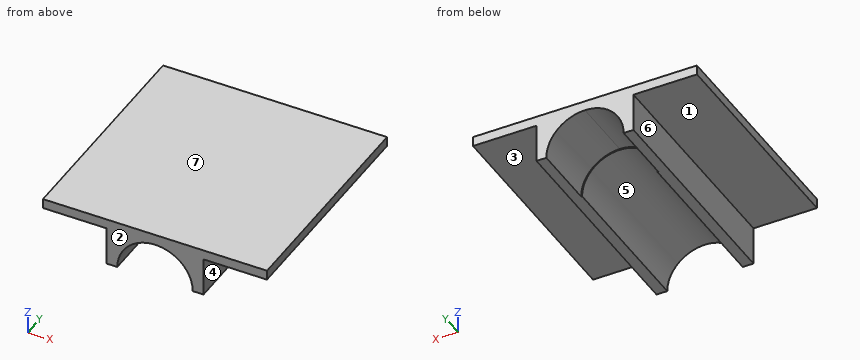
from build123d import *

# Parameters (mm, degrees)
BOSS_EXTRUDE4_DEPTH = 51.39
BOSS_EXTRUDE5_DEPTH = 72.39


with BuildPart() as part:
    # Sketch1 → Boss-Extrude4 (new body)
    with BuildSketch(Plane(origin=(0, 0, 0), x_dir=(1, 0, 0), z_dir=(0, 1, 0))):
        with BuildLine():
            ThreePointArc((18.7283116, 30.198170271), (6.5283116, 17.99817027), (-5.6716884, 30.198170271))
            Line((-5.6716884, 30.198170271), (-9.146688396, 30.198170271))
            Line((-9.146688396, 30.198170271), (-9.146688396, 17.698170271))
            Line((-9.146688396, 17.698170271), (-29.681604426, 17.698170271))
            Line((-29.681604426, 17.698170271), (-29.681604426, 14.523170271))
            Line((-29.681604426, 14.523170271), (42.719057074, 14.523170271))
            Line((42.719057074, 14.523170271), (42.719057074, 17.698170271))
            Line((42.719057074, 17.698170271), (22.203311604, 17.698170271))
            Line((22.203311604, 17.698170271), (22.203311604, 30.198170271))
            Line((22.203311604, 30.198170271), (18.7283116, 30.198170271))
        make_face()
    extrude(amount=BOSS_EXTRUDE4_DEPTH)

    # Sketch1_9 → Boss-Extrude5 (add)
    with BuildSketch(Plane(origin=(0, 0, 0), x_dir=(1, 0, 0), z_dir=(0, 1, 0))):
        Polygon((22.203311604, 17.698170271), (6.528311562, 17.698170271), (-9.146688396, 17.698170271), (-29.681604426, 17.698170271), (-29.681604426, 14.523170271), (42.719057074, 14.523170271), (42.719057074, 17.698170271), align=None)
        with BuildLine():
            ThreePointArc((19.028311604, 30.198170271), (15.367146354, 21.359335491), (6.528311562, 17.698170271))
            Line((6.528311562, 17.698170271), (22.203311604, 17.698170271))
            Line((22.203311604, 17.698170271), (22.203311604, 30.198170271))
            Line((22.203311604, 30.198170271), (19.028311604, 30.198170271))
        make_face()
        with BuildLine():
            ThreePointArc((6.528311562, 17.698170271), (-2.310523175, 21.359335521), (-5.971688396, 30.198170271))
            Line((-5.971688396, 30.198170271), (-9.146688396, 30.198170271))
            Line((-9.146688396, 30.198170271), (-9.146688396, 17.698170271))
            Line((-9.146688396, 17.698170271), (6.528311562, 17.698170271))
        make_face()
    extrude(amount=BOSS_EXTRUDE5_DEPTH)


solid = part.part
Design review of the part built by this model. Coordinates are the model's own, in mm. Face numbers are marked on the shaded views. A direction names the side the tool comes from. Give positions to 0.01 mm unless a question says otherwise; leave off trailing zeros. Order: outer loops, then holes, each group sorted by start corner. A loop starts at its lowest first (then second) coordinate and runs counter-clockwise, first axis right, second up. Notation, with made-up numbers: (-13.75, 34) - (28.25, 34) arc R17 cw to (28.25, 57) - close; hole circle Ø4 at (28, -21.5). An arc over 180 degrees is marked (long way). Write item = value, one per line. Start each with the question number.
Q1. To check wall thickness, follow L1, parallel to Z at x = -21.5, y = 7; L2, parallel to X at y = 21, z = -23.5; L3, parallel to X at y = 52, z = -20.5. State the ranges of each line that lie inside material, in increasing order. Write a range as from..to.
Q2. We need section C-C on z = -20.5. State the section outline as (x, y) points, plus the area to 3 significant figures.
Q3. We need section A-A on z = -26.75. State the section outline as (x, y) points.
Q4. Mouldability with a two-part tool opening along X and no side actions: class the marked faces 4, 5, 6 and 7 as released by +X, released by -X, zero draft, split by the parting line, or undercut.
Q5. We need section B-B on y = 55. State the section outline as (x, z) points.
Q6. We need section D-D on x = 17.5. State the section outline as (y, z) points, plus the area to 3 significant figures.
Q7. Clearance check with flat-ended pins moving along their axes: pin 1 Ø1 at (y, z) = (19.5, -23.5) entering from +X; pin 2 Ø1 at (y, z) = (52.5, -25) entering from -X; pin 3 Ø10.5 at (x, y) = (-17, 48.5) entering from -Z. State where each tip first meets the part, or that it passes through.
Q8. Tool access review of the marked faces 1, 2 and 3: name each direction out of +Z, -Z, +X, -X, +Y, -Y from which nothing blocks a thin tool from reaching the whole face with its end or side.
Working result:
q1.L1 = -17.7..-14.52
q1.L2 = -9.15..-3.67, 16.73..22.2
q1.L3 = -9.15..-1.36, 14.41..22.2
q2.outline = (-9.15, 0) - (-0.87, 0) - (-0.87, 51.39) - (-1.36, 51.39) - (-1.36, 72.39) - (-9.15, 72.39) - close; (13.93, 0) - (22.2, 0) - (22.2, 72.39) - (14.41, 72.39) - (14.41, 51.39) - (13.93, 51.39) - close
q2.area = 1,180 mm²
q3.outline = (-9.15, 0) - (-5.17, 0) - (-5.17, 51.39) - (-5.49, 51.39) - (-5.49, 72.39) - (-9.15, 72.39) - close; (18.23, 0) - (22.2, 0) - (22.2, 72.39) - (18.54, 72.39) - (18.54, 51.39) - (18.23, 51.39) - close
q4.face_4 = released by +X
q4.face_5 = undercut
q4.face_6 = released by -X
q4.face_7 = zero draft
q5.outline = (-29.68, -17.7) - (-9.15, -17.7) - (-9.15, -30.2) - (-5.97, -30.2) arc R12.5 cw to (19.03, -30.2) - (22.2, -30.2) - (22.2, -17.7) - (42.72, -17.7) - (42.72, -14.52) - (-29.68, -14.52) - close
q6.outline = (0, -24.86) - (51.39, -24.86) - (51.39, -24.21) - (72.39, -24.21) - (72.39, -14.52) - (0, -14.52) - close
q6.area = 735 mm²
q7.pin_1 = 22.2
q7.pin_2 = -9.15
q7.pin_3 = -17.7
q8.face_1 = -Z, -X, +Y, -Y
q8.face_2 = +Z, -Z, +X, -X, -Y
q8.face_3 = -Z, +X, +Y, -Y
